Source: three-view drawing plus pictorial views. Frame: mm from the lowest corner of the part. A direction names the side the tool comes from. Give positions to 0.01 mm unless a question says otherwise; leave off trailing zeros. Order: outer loops, then holes, each group sorted by start corner. A loop starts at its lowest first (then second) coordinate and runs counter-clockwise, first axis right, second up. Notation, with made-up numbers: M 21.25,66 L 79.25,66 A18 ccw 79.25,87 Z; hole C 14,52 d9. An arc over 180 degrees is marked long. Use CSV: the item, a comma, the result in double quotes. Start each with the question number.
1. Section query C-C, the plane x = 23.5. Return the cut outline in (y, z) (1 decimal).
2. Pin query (flat end, axial travel): P1, Ø9.5, axis at x = 12.83, y = 11.11, coming from the +Z side; P2, Ø10, axis at x = 18.5, z = 40, coming from the -Y side; P3, Ø3, axis at y = 11.5, z = 18.5, coming from the +X side; P4, Ø2, axis at y = 4.5, z = 14, coming from the -X side. Return the tip coordinate at first contact, or that it passes through.
3. Section query A-A, the plane z = 36.5. Return the cut outline in (x, y) (1 decimal).
4. Reachability of the marked faces 1 and 2 from +Z, -Z, +X, -X, +Y, -Y: full face, straight path, thin tool, end or side. Return the list, or none.
5. Section query B-B, the plane z = 22. Return the cut outline in (x, y) (1 decimal), plus the area to 3 significant figures.
6. Mould query, pull axis X, two halves, no side actions, for the marked faces 3, 4 and 5. Classes: released by +X, released by -X, zero draft, split by the parting line, or undercut.
7. Line query: line 1 along Y through (x, z) = (6.75, 13) (1 decimal); line 2 along X through (y, z) = (15.75, 35) (1 decimal); line 3 along Y through (x, z) = (12.75, 20.5) (1 decimal). Output: solid intervals per line, ascending. Write a range as [from, to].
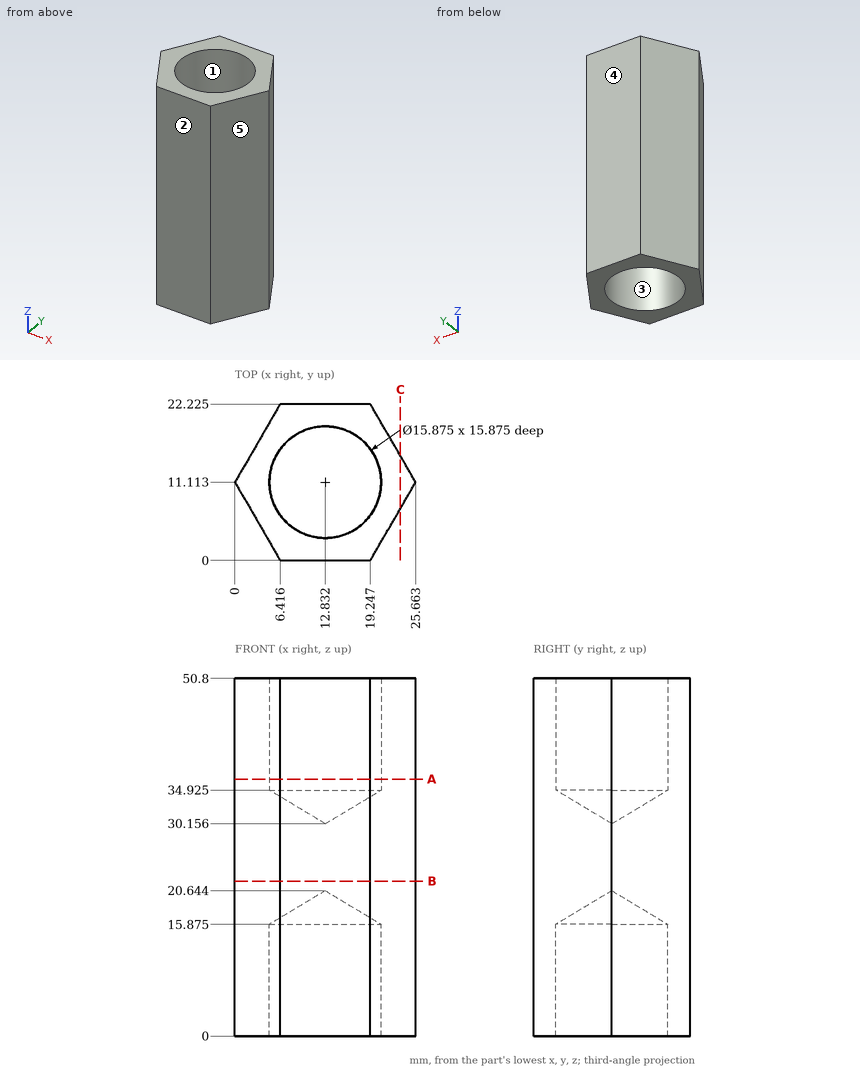
Result set:
1,outline,"M 7.4,0 L 14.9,0 L 14.9,50.8 L 7.4,50.8 Z"
2,P1,"z = 33.01"
2,P2,"y = 0"
2,P3,"x = 25.66"
2,P4,"x = 3.24"
3,outline,"M 0,11.1 L 6.4,0 L 19.2,0 L 25.7,11.1 L 19.2,22.2 L 6.4,22.2 Z; hole C 12.8,11.1 d15.9"
4,face 1,"+Z"
4,face 2,"+Z, -Z, +X, -X, -Y"
5,outline,"M 0,11.1 L 6.4,0 L 19.2,0 L 25.7,11.1 L 19.2,22.2 L 6.4,22.2 Z"
5,area,"428 mm2"
6,face 3,"undercut"
6,face 4,"zero draft"
6,face 5,"released by +X"
7,line 1,"[0, 6], [16.2, 22.2]"
7,line 2,"[2.7, 6.4], [19.3, 23]"
7,line 3,"[0, 10.9], [11.3, 22.2]"
